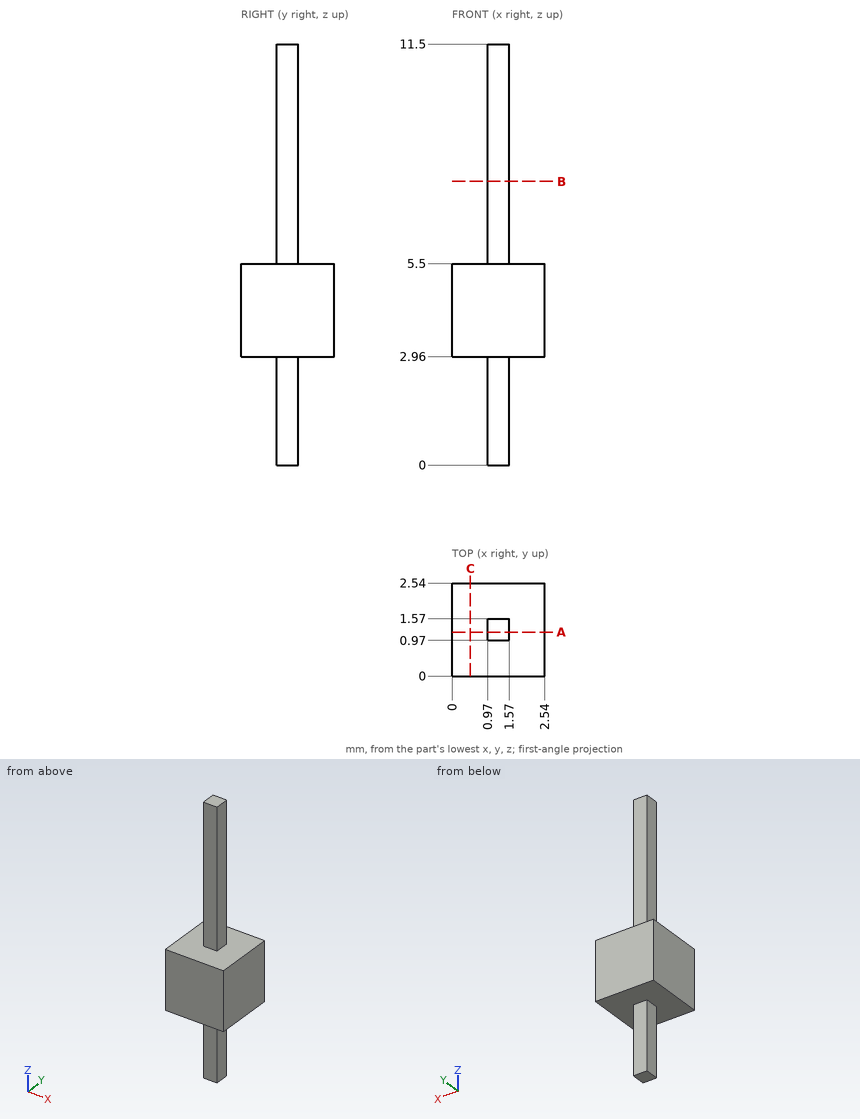
For this review, use the dimensioned drawing (mm, ordinates from the lowest corner) and the shaded views. Round coordinates to 2 decimals unless told otherwise and drop trailing zeros. Write each loop counter-clockwise with the first axis right and the second up, starting at its lowest first coordinate (ties: lowest second). Pieces come first, ordered by that corner, then holes. Notation, with made-up numbers: (55, 27.5) -> (59, 27.5) arc R12 cw to (59, 32.5) -> close; hole circle Ø2 at (-31.5, 87.25). An arc over 180 degrees is marked (long way). Use CSV: the item, a comma, the result in double quotes.
(1) Clearance check with flat-ended pins moving along their axes: P1, Ø0.7, axis at x = 1.5, z = 1.5, coming from the +Y side; P2, Ø0.5, axis at y = 1, z = 1, coming from the +X side; P3, Ø0.7, axis at x = 1, z = 8, coming from the -Y side. State where each tip first meets the part, or that it passes through.
Computed values:
P1,"y = 1.57"
P2,"x = 1.57"
P3,"y = 0.97"
(2) Consider section B-B, the plane z = 7.75. Give the boundary of the cut face in (x, y), plus the area to 3 significant figures.
Computed values:
outline,"(0.97, 0.97) -> (1.57, 0.97) -> (1.57, 1.57) -> (0.97, 1.57) -> close"
area,"0.360 mm²"
(3) Consider section C-C, the plane x = 0.5. Give the boundary of the cut face in (y, z), plus the area to 3 significant figures.
Computed values:
outline,"(0, 2.96) -> (2.54, 2.96) -> (2.54, 5.5) -> (0, 5.5) -> close"
area,"6.45 mm²"
(4) To check wall thickness, follow L1, parallel to Z at x = 1.95, y = 0.3; L2, parallel to Y at x = 1.4, z = 7.25. State the ranges of each line that lie inside material, in increasing order. Write a range as [from, to].
Computed values:
L1,"[2.96, 5.5]"
L2,"[0.97, 1.57]"
(5) Consider section A-A, the plane y = 1.2. Give the boundary of the cut face in (x, z).
Computed values:
outline,"(0, 2.96) -> (0.97, 2.96) -> (0.97, 0) -> (1.57, 0) -> (1.57, 2.96) -> (2.54, 2.96) -> (2.54, 5.5) -> (1.57, 5.5) -> (1.57, 11.5) -> (0.97, 11.5) -> (0.97, 5.5) -> (0, 5.5) -> close"
